```python
from build123d import *

# Parameters (mm, degrees)
SKETCH1_W           = 25.4
SKETCH1_H           = 25.4
SKETCH1_W_2         = 19.05
SKETCH1_H_2         = 19.05
BOSS_EXTRUDE1_DEPTH = 152.4
SKETCH2_R           = 2.1828125
CUT_EXTRUDE1_DEPTH  = 156.02325632
SKETCH3_R           = 3.3734375
CUT_EXTRUDE2_DEPTH  = 154.94


with BuildPart() as part:
    # Sketch1 → Boss-Extrude1 (new body)
    with BuildSketch(Plane(origin=(0, 0, 0), x_dir=(1, 0, 0), z_dir=(0, 1, 0))):
        Rectangle(SKETCH1_W, SKETCH1_H)
        Rectangle(SKETCH1_W_2, SKETCH1_H_2, mode=Mode.SUBTRACT)
    extrude(amount=BOSS_EXTRUDE1_DEPTH)

    # Sketch2 → Cut-Extrude1 (cut, through all)
    with BuildSketch(Plane.XY.offset(12.7)):
        with Locations((0, 11.1125)):
            Circle(SKETCH2_R)
        with Locations((0, 36.5125)):
            Circle(SKETCH2_R)
    extrude(amount=-CUT_EXTRUDE1_DEPTH, mode=Mode.SUBTRACT)

    # Sketch3 → Cut-Extrude2 (cut)
    with BuildSketch(Plane(origin=(12.7, 0, 0), x_dir=(0, 0, -1), z_dir=(1, 0, 0))):
        with Locations((0, 133.35)):
            Circle(SKETCH3_R)
    extrude(amount=-CUT_EXTRUDE2_DEPTH, mode=Mode.SUBTRACT)


solid = part.part
```
Could you check a few things on this model? Use its own coordinates, in mm. A direction names the side the tool comes from. Give positions to 0.01 mm unless a question says otherwise; leave off trailing zeros. Order: outer loops, then holes, each group sorted by start corner. A loop starts at its lowest first (then second) coordinate and runs counter-clockwise, first axis right, second up.
Q1. Suppose I cut it at C-C, the plane z = 8. Write out the boundary of the cut face in (x, y) (3 decimals).
Q2. Suppose I cut it at A-A, the plane y = 133.35. Write out the boundary of the cut face in (x, z) (3 decimals), and give its area (3 significant figures).
Q3. We'd pull the mould along X, two halves only. Please class faces 1 (the flat face through (9.525, 75, 0)), 2 (the flat face through (12.7, 75, 0)), 3 (the cylindrical face through (1.007, 34.576, 11.135)), 4 (the flat face through (-12.7, 75, 0)): +X half, -X half, draft (parallel to the pull), parting line (faces both ways), or undercut.
Q4. I'm going to push a flat-ended pin straight in: P1, Ø3.5, axis at x = 0, y = 11.11, coming from the -Z side. Where does the tip first touch, or does it pass through?
Q5. Suppose I cut it at D-D, the plane x = 6. Write out the boundary of the cut face in (y, z) (3 decimals), and give its area (3 significant figures).
Q6. For faces 5 (the flat face through (0, 75, -9.525)), 6 (the cylindrical face through (1.007, 34.576, -11.09)), which set-ups out of +Z, -Z, +X, -X, +Y, -Y let a thin tool reach every point of the face, with its end or its side?
Q7. If I drill on line 1 along Y through (x, z) = (0, -11); line 2 along X through (y, z) = (92, 2.25) (3 decimals), over which ranges is the centre line in solid material (lowest first)?
Q8. Suppose I cut it at B-B, the plane x = 0. Write out the boundary of the cut face in (y, z) (3 decimals).
Solution:
1. outline: (-12.7, 0) - (-9.525, 0) - (-9.525, 152.4) - (-12.7, 152.4) - close; (9.525, 0) - (12.7, 0) - (12.7, 152.4) - (9.525, 152.4) - close
2. outline: (-12.7, -12.7) - (12.7, -12.7) - (12.7, -3.373) - (9.525, -3.373) - (9.525, -9.525) - (-9.525, -9.525) - (-9.525, -3.373) - (-12.7, -3.373) - close; (-12.7, 3.373) - (-9.525, 3.373) - (-9.525, 9.525) - (9.525, 9.525) - (9.525, 3.373) - (12.7, 3.373) - (12.7, 12.7) - (-12.7, 12.7) - close
2. area: 239 mm2
3. face 1: undercut
3. face 2: +X half
3. face 3: undercut
3. face 4: -X half
4. P1: passes through
5. outline: (0, -12.7) - (152.4, -12.7) - (152.4, -9.525) - (0, -9.525) - close; (0, 9.525) - (152.4, 9.525) - (152.4, 12.7) - (0, 12.7) - close
5. area: 968 mm2
6. face 5: +Y, -Y
6. face 6: +Z, -Z
7. line 1: y = 0 to 8.93, 13.3 to 34.33, 38.7 to 152.4
7. line 2: x = -12.7 to -9.525, 9.525 to 12.7
8. outline: (0, -12.7) - (8.93, -12.7) - (8.93, -9.525) - (0, -9.525) - close; (0, 9.525) - (8.93, 9.525) - (8.93, 12.7) - (0, 12.7) - close; (13.295, -12.7) - (34.33, -12.7) - (34.33, -9.525) - (13.295, -9.525) - close; (13.295, 9.525) - (34.33, 9.525) - (34.33, 12.7) - (13.295, 12.7) - close; (38.695, -12.7) - (152.4, -12.7) - (152.4, -9.525) - (38.695, -9.525) - close; (38.695, 9.525) - (152.4, 9.525) - (152.4, 12.7) - (38.695, 12.7) - close
